Design review of the part built by this model. Coordinates are the model's own, in mm. Face numbers are marked on the shaded views. A direction names the side the tool comes from. Round coordinates to 2 decimals unless told otherwise and drop trailing zeros. Loops run counter-clockwise (first coordinate to the right, second up) from the corner with the lowest first, then second, coordinate; pieces in that order, holes last. Notation, with made-up numbers: (35.5, 13.5) - (44.5, 13.5) arc R18 cw to (44.5, 20.5) - close; hole circle Ø9 at (84, -7). An arc over 180 degrees is marked (long way). Use one line per item in the form item = value. Start each with the question number.
(1) We need section A-A, the plane x = 0. Write out the cut boundary in (y, z) (3 decimals), then the cut area to 3 significant figures.
(2) The part is to be moulded in two halves that separate along Z. For the marked faces 3 and 4, say which applies: released by +Z, released by -Z, zero draft, split by the parting line, or undercut.
(3) Wall thickness on probe 1 along Z at (x, y) = (13, 10); probe 2 along Z at (x, y) = (17.5, -6); probe 3 along Y at (x, z) = (8, 34): over which ranges is each line inside the solid? List them lowest first. Write a range as [from, to].
(4) We need section C-C, the plane z = 38. Write out the cut boundary in (x, y).
(5) Machinability: for the marked faces 1 and 2, which of the approach directions +Z, -Z, +X, -X, +Y, -Y give a long, thin tool a straight path to every point of the face, cutting with its end or side? Answer none if there is none.
(6) For pin 1 (6 mm diameter, centred on x = 13, z = 38, fed in from +Y); pin 2 (4 mm diameter, centred on y = 5, z = 40.5, fed in from -X); pin 3 (6 mm diameter, centred on x = -4, z = 27, fed in from +Y), all flat-tipped, find the tip position at first contact; note any pin that passes through.
(7) We need section D-D, the plane z = 34. Write out the cut boundary in (x, y).
from build123d import *

# Parameters (mm, degrees)
SKETCH058_W  = 38.59
SKETCH058_H  = 38.59
PAD041_DEPTH = 20.7
PAD041_TAPER = 2
SKETCH059_R  = 17.645
PAD042_DEPTH = 12.8
PAD042_TAPER = 1.5
FILLET_R     = 1
FILLET003_R  = 5
FILLET004_R  = 0.5


with BuildPart() as part:
    # Sketch058 → Pad041 (new body)
    with BuildSketch(Plane.XY):
        Rectangle(SKETCH058_W, SKETCH058_H)
    extrude(amount=PAD041_DEPTH, taper=PAD041_TAPER)

    # Sketch059 (on Face6 of Pad041) → Pad042 (join)
    with BuildSketch(Plane.XY.offset(20.7)):
        Circle(SKETCH059_R)
    extrude(amount=PAD042_DEPTH, taper=PAD042_TAPER)

    # Fillet
    fillet_edges = [part.edges().sort_by_distance(p)[0] for p in [
        (-17.30982, 0, 33.5),
    ]]
    fillet(fillet_edges, radius=FILLET_R)

    # Fillet003
    fillet003_edges = [part.edges().sort_by_distance(p)[0] for p in [
        (18.93357, -18.93357, 10.35),
        (18.93357, 18.93357, 10.35),
        (-18.93357, 18.93357, 10.35),
        (-18.93357, -18.93357, 10.35),
    ]]
    fillet(fillet003_edges, radius=FILLET003_R)

    # Fillet004
    fillet004_edges = [part.edges().sort_by_distance(p)[0] for p in [
        (0, -18.57214, 20.7),
        (-17.108935, -17.108935, 20.7),
        (-18.57214, 0, 20.7),
        (18.57214, 0, 20.7),
        (17.108935, 17.108935, 20.7),
        (0, 18.57214, 20.7),
        (17.108935, -17.108935, 20.7),
        (-17.108935, 17.108935, 20.7),
    ]]
    fillet(fillet004_edges, radius=FILLET004_R)


with BuildPart() as part_1:
    # Body023 placement: moved
    add(part.part.moved(Location((0, 0, 11))))


solid = part_1.part
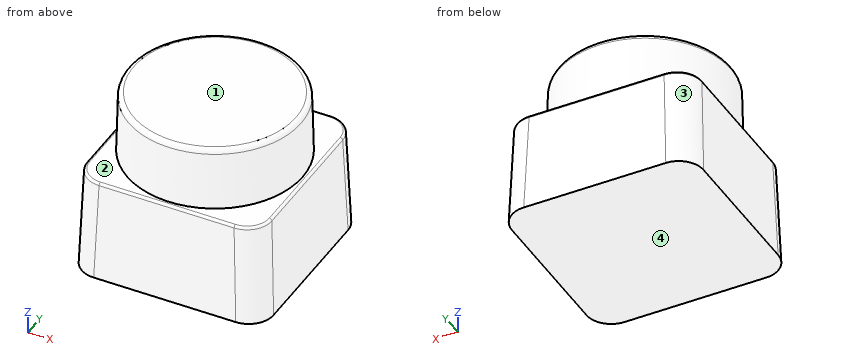
Data:
q1.outline = (-19.295, 11) - (19.295, 11) - (18.589, 31.217) arc R0.5 ccw to (18.089, 31.7) - (17.645, 31.7) - (17.335, 43.526) arc R1 ccw to (16.336, 44.5) - (-16.336, 44.5) arc R1 ccw to (-17.335, 43.526) - (-17.645, 31.7) - (-18.089, 31.7) arc R0.5 ccw to (-18.589, 31.217) - close
q1.area = 1,230 mm^2
q2.face_3 = released by +Z
q2.face_4 = released by -Z
q3.probe_1 = [11, 44.5]
q3.probe_2 = [11, 31.7]
q3.probe_3 = [-15.66, 15.66]
q4.outline = circle Ø34.96 at (0, 0)
q5.face_1 = +Z, +X, -X, +Y, -Y
q5.face_2 = +Z
q6.pin_1 = 14.34
q6.pin_2 = -17.16
q6.pin_3 = 18.84
q7.outline = circle Ø35.17 at (0, 0)
